Autodesk Inventor part; units mm, degrees
ref_plane "YZ Plane" through (0, 0, 0) normal (1, 0, 0) x (0, 1, 0)
ref_plane "XZ Plane" through (0, 0, 0) normal (0, 1, 0) x (-1, 0, 0)
ref_plane "XY Plane" through (0, 0, 0) normal (0, 0, 1) x (1, 0, 0)
sketch "Sketch1" plane through (0, 0, 0) normal (0, 0, 1) x (1, 0, 0)
  line L0 (0, 0) -> (60, 0)
  line L1 (60, 0) -> (60, -60)
  line L2 (60, -60) -> (0, -60)
  line L3 (0, -60) -> (0, 0)
  dimension "d0" = 60
  dimension "d1" = 60
extrude "Extrusion1" add sketch "Sketch1" against normal blind 15
sketch "Sketch2" plane through (0, 0, 0) normal (0, 0, 1) x (1, 0, 0)
  line L0 (0, 0) -> (60, 0)
  line L1 (0, -60) -> (0, 0)
  line L2 (60, -60) -> (0, -60)
  line L3 (60, 0) -> (60, -60)
  circle A0 centre (5, -5) radius 2.15
  circle A1 centre (55, -5) radius 2.15
  circle A2 centre (55, -55) radius 2.15
  circle A3 centre (5, -55) radius 2.15
  dimension "d5" = 4.3
  dimension "d6" = 4.3
  dimension "d7" = 4.3
  dimension "d8" = 4.3
  dimension "d9" = 50
  dimension "d10" = 50
  dimension "d11" = 5
  dimension "d12" = 5
extrude "Extrusion2" cut sketch "Sketch2" against normal up to next contours A0 | A1 | A2 | A3
sketch "Sketch3" plane through (0, 0, 0) normal (0, 0, 1) x (1, 0, 0)
  circle A0 centre (55, -55) radius 2.15
  circle A1 centre (5, -5) radius 2.15
  circle A2 centre (55, -5) radius 2.15
  circle A3 centre (5, -55) radius 2.15
  line L0 (0, 0) -> (60, 0)
  line L1 (0, -60) -> (0, 0)
  line L2 (60, -60) -> (0, -60)
  line L3 (60, 0) -> (60, -60)
  line L4 (15.0313, -2) -> (44.9687, -2)
  line L5 (2, -44.9687) -> (2, -15.0313)
  line L6 (44.9687, -58) -> (15.0313, -58)
  line L7 (58, -15.0313) -> (58, -44.9687)
  arc A4 (15.0313, -2) -> (2, -15.0313) centre (30, -30) ccw
  arc A5 (2, -44.9687) -> (15.0313, -58) centre (30, -30) ccw
  arc A6 (44.9687, -58) -> (58, -44.9687) centre (30, -30) ccw
  arc A7 (58, -15.0313) -> (44.9687, -2) centre (30, -30) ccw
  dimension "d23" = 360
  dimension "d16" = 60
  dimension "d17" = 30
  dimension "d18" = 30
  dimension "d20" = 2
extrude "Extrusion3" cut sketch "Sketch3" against normal up to next contours L4 A7 L7 A6 L6 A5 L5 A4
fillet "Fillet2" radius 3.175 4 edges at (0, 0, -7.5) (0, -60, -7.5) (60, -60, -7.5) (60, 0, -7.5)
equation "\"d1\" = d0"
equation "\"d6\" = d5"
equation "\"d7\" = d5"
equation "\"d8\" = d5"
equation "\"d10\" = d9"
equation "\"d12\" = d11"
equation "\"d17\" = 0.5 * d16"
equation "\"d18\" = d17"
properties part number "60mm Fan Footprint" material "ABS Plastic"
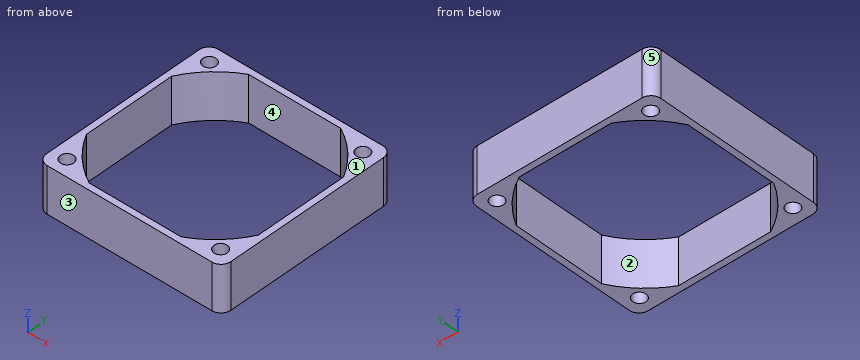
Read the model definition and answer for the solid it produces. Units are mm, in the model's axes. Face numbers are marked on the shaded views. A direction names the side the tool comes from. Round coordinates to 2 decimals unless told otherwise and drop trailing zeros. Write each loop counter-clockwise with the first axis right and the second up, starting at its lowest first coordinate (ties: lowest second). Pieces come first, ordered by that corner, then holes. Notation, with made-up numbers: (50.25, 5) - (109.25, 5) arc R25 cw to (109.25, 42) - close; hole circle Ø5 at (78.5, -19.5). An arc over 180 degrees is marked (long way). Use a Markdown table: item, result.
(1) The part is cut by section B-B (x = 17). Write down the section's boundary in (y, z).
Reported:
| item | result |
|---|---|
| outline | (-60, -15) - (-58, -15) - (-58, 0) - (-60, 0) - close; (-2, -15) - (0, -15) - (0, 0) - (-2, 0) - close |
(2) The part is cut by section A-A (z = -1). Write down the section's boundary in (x, y) (3 decimals), then the cut area to 3 significant figures.
Reported:
| item | result |
|---|---|
| outline | (0, -56.825) arc R3.175 ccw to (3.175, -60) - (56.825, -60) arc R3.175 ccw to (60, -56.825) - (60, -3.175) arc R3.175 ccw to (56.825, 0) - (3.175, 0) arc R3.175 ccw to (0, -3.175) - close; hole (2, -44.969) arc R31.75 ccw to (15.031, -58) - (44.969, -58) arc R31.75 ccw to (58, -44.969) - (58, -15.031) arc R31.75 ccw to (44.969, -2) - (15.031, -2) arc R31.75 ccw to (2, -15.031) - close; hole circle Ø4.3 at (5, -55); hole circle Ø4.3 at (5, -5); hole circle Ø4.3 at (55, -55); hole circle Ø4.3 at (55, -5) |
| area | 669 mm2 |
(3) The part is cut by section C-C (y = -46). Write down the section's boundary in (x, z).
Reported:
| item | result |
|---|---|
| outline | (0, -15) - (2.58, -15) - (2.58, 0) - (0, 0) - close; (57.42, -15) - (60, -15) - (60, 0) - (57.42, 0) - close |
(4) Straight lines are drawn through the part: line 1 along Y through (x, z) = (23.5, -12.75); line 2 along Y through (x, z) = (54.5, -12.75); line 3 along X through (y, z) = (-17.5, -4). For each, find the intervals that lie inside material, in ascending order. Write a range as [from, to].
Reported:
| item | result |
|---|---|
| line 1 | [-60, -58], [-2, 0] |
| line 2 | [-60, -57.09], [-52.91, -50.19], [-9.81, -7.09], [-2.91, 0] |
| line 3 | [0, 2], [58, 60] |
(5) Which of the six approach directions +Z, -Z, +X, -X, +Y, -Y give full straight-line access (tool end or side, diameter ignored) to the marked faces 1 and 2?
Reported:
| item | result |
|---|---|
| face 1 | +Z, +X, -X, +Y, -Y |
| face 2 | +Z, -Z |
(6) The part is cut by section D-D (y = -55). Write down the section's boundary in (x, z), then the cut area to 3 significant figures.
Reported:
| item | result |
|---|---|
| outline | (0, -15) - (2.85, -15) - (2.85, 0) - (0, 0) - close; (7.15, -15) - (10.43, -15) - (10.43, 0) - (7.15, 0) - close; (49.57, -15) - (52.85, -15) - (52.85, 0) - (49.57, 0) - close; (57.15, -15) - (60, -15) - (60, 0) - (57.15, 0) - close |
| area | 184 mm2 |
(7) The mould has two halves that part along X. Classify the marked faces 3, 4 and 5: released by +X, released by -X, zero draft, split by the parting line, or undercut.
Reported:
| item | result |
|---|---|
| face 3 | zero draft |
| face 4 | undercut |
| face 5 | released by -X |
